from build123d import *

# Parameters (mm, degrees)
CYLINDER007_R     = 11
CYLINDER007_DEPTH = 22
CYLINDER006_R     = 30.5
CYLINDER006_DEPTH = 22


with BuildPart() as cylinder007:
    # Cylinder007 → Cylinder007 (new body)
    with BuildSketch(Plane.XY):
        Circle(CYLINDER007_R)
    extrude(amount=CYLINDER007_DEPTH)


with BuildPart() as obj1:
    # Cylinder006 → Cylinder006 (new body)
    with BuildSketch(Plane.XY):
        Circle(CYLINDER006_R)
    extrude(amount=CYLINDER006_DEPTH)

    # Cut006: cut Cylinder007
    add(cylinder007.part, mode=Mode.SUBTRACT)


with BuildPart() as obj1_1:
    # Cut006 placement: moved
    add(obj1.part.moved(Location((51.5, 17, 2))))


solid = obj1_1.part
Could you check a few things on this model? Use its own coordinates, in mm. Round coordinates to 2 decimals unless told otherwise and drop trailing zeros. Loops run counter-clockwise (first coordinate to the right, second up) from the corner with the lowest first, then second, coordinate; pieces in that order, holes last. Notation, with made-up numbers: (58, -12.5) - (85, -12.5) arc R19 ccw to (85, 0.5) - close; hole circle Ø5 at (28, -23.75). An arc over 180 degrees is marked (long way). Write item = value, one per line.
1) Imagine slicing it at B-B (y = 17). Please give me the cut outline in (x, z).
Computed:
outline = (21, 2) - (40.5, 2) - (40.5, 24) - (21, 24) - close; (62.5, 2) - (82, 2) - (82, 24) - (62.5, 24) - close
2) Imagine slicing it at C-C (z = 13.75). Please give me the cut outline in (x, y).
Computed:
outline = circle Ø61 at (51.5, 17); hole circle Ø22 at (51.5, 17)
3) Imagine slicing it at A-A (x = 51.5). Please give me the cut outline in (y, z), and give its area (3 significant figures).
Computed:
outline = (-13.5, 2) - (6, 2) - (6, 24) - (-13.5, 24) - close; (28, 2) - (47.5, 2) - (47.5, 24) - (28, 24) - close
area = 858 mm2
4) I'm going to push flat-ended pins straight in: P1, Ø1.5, axis at x = 61.5, z = 11, coming from the +Y side; P2, Ø3, axis at y = 24, z = 20.5, coming from the -X side; P3, Ø3, axis at x = 66.5, z = 12, coming from the +Y side. Where does each tip first touch, or does it pass through?
Computed:
P1 = 46.06
P2 = 21.5
P3 = 44.35
5) Imagine slicing it at D-D (y = 31). Please give me the cut outline in (x, z).
Computed:
outline = (24.4, 2) - (78.6, 2) - (78.6, 24) - (24.4, 24) - close
6) If we mould it in two halves opening along Y, with no side actions, what happens to faces 1 (the cylindrical face through (49.12, 6.26, 12.85)), 2 (the flat face through (51, 4, 24)), 3 (the cylindrical face through (67.897, 42.718, 12.846))? For each: pulls with the +Y half, pulls with the -Y half, needs draft (parallel to the pull), parting line crosses it, or undercut.
Computed:
face_1 = undercut
face_2 = needs draft
face_3 = parting line crosses it
7) I need wall thicknesses on line 1 along Y through (x, z) = (51.5, 10.25); line 2 along Y through (x, z) = (44.5, 22); line 3 along X through (y, z) = (27, 16.5). Which ranges of each line are inside material? Lowest first, please. Write a range as from..to.
Computed:
line_1 = -13.5..6, 28..47.5
line_2 = -12.69..8.51, 25.49..46.69
line_3 = 22.69..46.92, 56.08..80.31
